The listing builds one solid part. Answer for the finished solid, in the listing's coordinates (mm). Face numbers are marked on the shaded views. A direction names the side the tool comes from. Round coordinates to 2 decimals unless told otherwise and drop trailing zeros. Write each loop counter-clockwise with the first axis right and the second up, starting at its lowest first coordinate (ties: lowest second). Pieces come first, ordered by that corner, then holes.
Item 1: For a pull along X with two mould halves and no side action, classify the marked faces 1, 2, 3 and 4 as +X half, -X half, draft (parallel to the pull), parting line (faces both ways), or undercut.
Item 2: Find section A-A on y = 0. Give the vertices of the cut face in (x, z), then the cut area to 3 significant figures.
Item 3: A tool of negligible diameter and unlimited length cuts with its end or side. For the marked faces 5 and 6, from which of +Z, -Z, +X, -X, +Y, -Y can it reach the whole face along a straight path? Write none if from no direction.
Item 4: Find section D-D on y = -17. Give the vertices of the cut face in (x, z).
Item 5: Find the intervals of material crossed by probe 1 along Y at (x, z) = (18, 37); probe 2 along Z at (x, y) = (51.75, 0); probe 3 along X at (y, z) = (-16.5, 8), in increasing order.
Item 6: Find section B-B on z = 6.5. Give the vertices of the cut face in (x, y), then the cut area to 3 significant figures.
Item 7: Each of these flat-tipped pins is pushed along its axis until it touches: pin 1 (3 mm diameter, centred on x = 7, y = -19.5, fed in from +Z); pin 2 (25 mm diameter, centred on y = 0, z = 28.99, fed in from +X). Where does it stop, or does it pass through?
Item 8: Find section C-C on x = 47.5. Give the vertices of the cut face in (y, z), then the cut area to 3 significant figures.
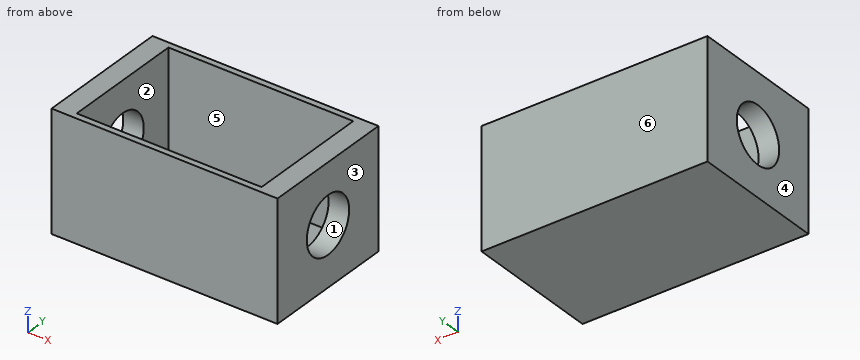
```python
from build123d import *

# Parameters (mm, degrees)
F0_W     = 110
F0_H     = 66
F1_DEPTH = 58
F2_W     = 90
F2_H     = 60
F3_DEPTH = 55
F5_R     = 13.843831
F6_DEPTH = 115


with BuildPart() as f1:
    # F0 (on Top) → F1 (new body)
    with BuildSketch(Plane.XY):
        Rectangle(F0_W, F0_H)
    extrude(amount=F1_DEPTH)

    # F2 (on face) → F3 (cut)
    with BuildSketch(Plane.XY.offset(58)):
        Rectangle(F2_W, F2_H)
    extrude(amount=-F3_DEPTH, mode=Mode.SUBTRACT)

    # F5 (on face) → F6 (cut)
    with BuildSketch(Plane(origin=(-55, 0, 0), x_dir=(0, -1, 0), z_dir=(-1, 0, 0))):
        with Locations((0, 28.994452)):
            Circle(F5_R)
    extrude(amount=-F6_DEPTH, mode=Mode.SUBTRACT)


solid = f1.part
```
Check values:
1. face 1: draft
1. face 2: undercut
1. face 3: +X half
1. face 4: -X half
2. outline: (-55, 0) - (55, 0) - (55, 15.15) - (45, 15.15) - (45, 3) - (-45, 3) - (-45, 15.15) - (-55, 15.15) - close; (-55, 42.84) - (-45, 42.84) - (-45, 58) - (-55, 58) - close; (45, 42.84) - (55, 42.84) - (55, 58) - (45, 58) - close
2. area: 876 mm2
3. face 5: +Z
3. face 6: +Z, -Z, +X, -X, +Y
4. outline: (-55, 0) - (55, 0) - (55, 58) - (45, 58) - (45, 3) - (-45, 3) - (-45, 58) - (-55, 58) - close
5. probe 1: y = -33 to -30, 30 to 33
5. probe 2: z = 0 to 15.15, 42.84 to 58
5. probe 3: x = -55 to -45, 45 to 55
6. outline: (-55, -33) - (55, -33) - (55, 33) - (-55, 33) - close; hole (-45, -30) - (45, -30) - (45, 30) - (-45, 30) - close
6. area: 1,860 mm2
7. pin 1: stops at z = 3
7. pin 2: passes through
8. outline: (-33, 0) - (33, 0) - (33, 58) - (-33, 58) - close; hole circle Ø27.69 at (0, 28.99)
8. area: 3,230 mm2
